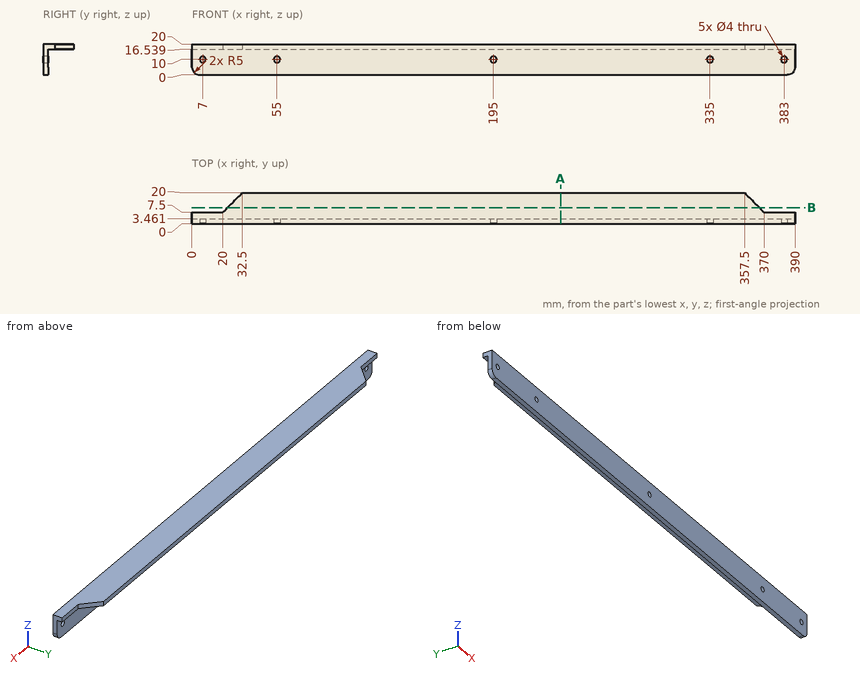
Here's the drawing with two shaded views (mm, measured from the low corner). I have some questions. Coordinates: 2 decimals unless noted, no trailing zeros. Order: outer loops, then holes, each group sorted by start corner. A loop starts at its lowest first (then second) coordinate and runs counter-clockwise, first axis right, second up. Notation, with made-up numbers: (67.25, 61.25) - (79.25, 61.25) arc R22 ccw to (79.25, 72.25) - close; hole circle Ø7 at (-9, 37). An arc over 180 degrees is marked (long way). Answer in a Markdown table with one row per item.
1. For pin 1 (2.5 mm diameter, centred on x = 383, z = 10, fed in from +Y); pin 2 (5 mm diameter, centred on x = 7, z = 10, fed in from +Y); pin 3 (10 mm diameter, centred on x = 157.5, y = 11.5, fed in from -Z); pin 4 (3 mm diameter, centred on x = 382, z = 19, fed in from +Y), each with a flat end and sliding along its axis, tell me the tip position at first contact or that it passes through.
Reply:
| item | result |
|---|---|
| pin 1 | passes through |
| pin 2 | stops at y = 3.46 |
| pin 3 | stops at z = 16.54 |
| pin 4 | stops at y = 7.5 |
2. If I drill on line 1 along X through (y, z) = (0.8, 10); line 2 along Z through (x, y) = (335, 2.8); line 3 along Y through (x, z) = (188, 6.5), over which ranges is the centre line in solid material (lowest first)?
Reply:
| item | result |
|---|---|
| line 1 | x = 0 to 5, 9 to 53, 57 to 193, 197 to 333, 337 to 381, 385 to 390 |
| line 2 | z = 0 to 8, 12 to 20 |
| line 3 | y = 0 to 3.46 |
3. Suppose I cut it at B-B (y = 10.5). Please give me the cut outline in (x, z), and give its area (3 significant figures).
Reply:
| item | result |
|---|---|
| outline | (23, 16.54) - (367, 16.54) - (367, 20) - (23, 20) - close |
| area | 1,190 mm^2 |
4. Suppose I cut it at A-A (x = 238.5). Please give me the cut outline in (y, z), and give its area (3 significant figures).
Reply:
| item | result |
|---|---|
| outline | (0, 0) - (3.46, 0) - (3.46, 16.54) - (20, 16.54) - (20, 20) - (0, 20) - close |
| area | 126 mm^2 |
